Autodesk Inventor part; units mm, degrees
ref_plane "YZ Plane" through (0, 0, 0) normal (1, 0, 0) x (0, 1, 0)
ref_plane "XZ Plane" through (0, 0, 0) normal (0, 1, 0) x (-1, 0, 0)
ref_plane "XY Plane" through (0, 0, 0) normal (0, 0, 1) x (1, 0, 0)
sketch "Sketch1" plane through (0, 0, 0) normal (0, 1, 0) x (-1, 0, 0)
  line L0 (87.5, 87.5) -> (-87.5, 87.5)
  line L1 (-87.5, 87.5) -> (-87.5, -87.5)
  line L2 (-87.5, -87.5) -> (87.5, -87.5)
  line L3 (87.5, -87.5) -> (87.5, 87.5)
  line L4 (87.5, 87.5) -> (-87.5, -87.5) construction
  line L5 (40, 40) -> (-40, 40) construction
  line L6 (-40, 40) -> (-40, -40) construction
  line L7 (-40, -40) -> (40, -40) construction
  line L8 (40, -40) -> (40, 40) construction
  line L9 (-40, 40) -> (40, -40) construction
  point P0 (0, 0)
  point P1 (0, 0)
  point P2 (0, 87.5)
  dimension "d0" = 175
  dimension "d1" = 175
  dimension "d2" = 80
  dimension "d3" = 80
extrude "Plate1" add sketch "Sketch1" along normal blind 3
sketch "Sketch2" plane through (0, 3, 0) normal (0, 1, 0) x (1, 0, 0)
  circle A0 centre (0, -63.75) radius 6
  line L0 (87.5, -87.5) -> (-87.5, -87.5)
  point P0 (0, 0)
  point P1 (0, -87.5)
  dimension "d7" = 23.75
  dimension "d8" = 12
extrude "Extrusion1" cut sketch "Sketch2" against normal blind 10
pattern_circular "Circular Pattern1" count 4 over 360 about axis through (0, -10, 0) along (0, 1, 0) of "Extrusion1"
equation "\"BendReliefWidth\" = Thickness"
equation "\"BendReliefDepth\" = 0.5 * Thickness"
equation "\"CornerReliefSize\" = 4 * Thickness"
equation "\"MinimumRemnant\" = 2 * Thickness"
equation "\"TransitionRadius\" = BendRadius"
equation "\"JacobiRadiusSize\" = BendRadius"
equation "\"GapSize\" = Thickness"
properties part number "MSC 127 flange frame heel" material "Stainless Steel"
Read the model definition and answer for the solid it produces. Units are mm, in the model's axes. Give positions to 0.01 mm unless a question says otherwise; leave off trailing zeros. Write each loop counter-clockwise with the first axis right and the second up, starting at its lowest first coordinate (ties: lowest second). Pieces come first, ordered by that corner, then holes. Notation, with made-up numbers: (80.5, 44.5) -> (107.5, 44.5) arc R14 cw to (107.5, 67.5) -> close; hole circle Ø6 at (48, -25). An arc over 180 degrees is marked (long way). Answer as a JSON object with one key per item and string values. Group by question number.
1) Consider L1, parallel to X at y = 1.8, z = 0; L2, parallel to X at y = 1.75, z = 63.75. Determine where each line is inside the solid, lowest interval first. Write a range as from..to.
2) This flat-tipped pin is pushed along its axis until it touches: P1, Ø9.5, axis at x = 63.75, z = 0, coming from the +Y side. Where does it stop, or does it pass through?
3) The mould has two halves that part along X. Classify faces 1 (the flat face through (1, 0, 1)), 2 (the cylindrical face through (-1.301, 1.521, 69.607)): +X half, -X half, draft (parallel to the pull), parting line (faces both ways), or undercut.
4) Find section C-C (x = -63.75). Write down the section's boundary in (y, z), and give its area (3 significant figures).
5) Find section A-A (x = 0). Write down the section's boundary in (y, z).
6) Find section B-B (z = -63.75). Write down the section's boundary in (x, y), and give its area (3 significant figures).
Values follow:
{
 "1": {"L1": "x = -87.5..-69.75, -57.75..57.75, 69.75..87.5", "L2": "x = -87.5..-6, 6..87.5"},
 "2": {"P1": "passes through"},
 "3": {"face 1": "draft", "face 2": "undercut"},
 "4": {"outline": "(0, -87.5) -> (3, -87.5) -> (3, -6) -> (0, -6) -> close; (0, 6) -> (3, 6) -> (3, 87.5) -> (0, 87.5) -> close", "area": "489 mm2"},
 "5": {"outline": "(0, -87.5) -> (3, -87.5) -> (3, -69.75) -> (0, -69.75) -> close; (0, -57.75) -> (3, -57.75) -> (3, 57.75) -> (0, 57.75) -> close; (0, 69.75) -> (3, 69.75) -> (3, 87.5) -> (0, 87.5) -> close"},
 "6": {"outline": "(-87.5, 0) -> (-6, 0) -> (-6, 3) -> (-87.5, 3) -> close; (6, 0) -> (87.5, 0) -> (87.5, 3) -> (6, 3) -> close", "area": "489 mm2"}
}
